Read the model definition and answer for the solid it produces. Units are mm, in the model's axes. Face numbers are marked on the shaded views. Coordinates: 2 decimals unless noted, no trailing zeros. Order: outer loops, then holes, each group sorted by start corner. A loop starts at its lowest first (then second) coordinate and runs counter-clockwise, first axis right, second up. Notation, with made-up numbers: (2.25, 43.25) -> (58.25, 43.25) arc R18 cw to (58.25, 75.25) -> close; hole circle Ø7 at (79, 65.25). An arc over 180 degrees is marked (long way). Answer as a JSON object with one key per item and string values. Group by question number.
1) Given pin 1 (3 mm diameter, centred on x = 16, y = 0, fed in from +Z); pin 2 (4 mm diameter, centred on x = -11.31, y = 11.31, fed in from -Z); pin 3 (4 mm diameter, centred on x = 17.5, z = 27.75, fed in from +Y); pin 4 (2.5 mm diameter, centred on x = -11.31, y = -11.31, fed in from +Z), each flat-ended and moving along its own axis, determine where each tip first touches the part or whether it passes through.
2) Consider L1, parallel to Y at x = 0, z = 19; L2, parallel to X at y = 12.5, z = 30; L3, parallel to X at y = 14, z = 26.5. Determine where each line is inside the solid, lowest interval first.
3) Determine the mould class of the marked faces 1, 2, 3 and 4 for opening direction X: released by +X, released by -X, zero draft, split by the parting line, or undercut.
4) Section B-B on y = 6.5 is taken. Count the separate pieces of the cut face and the enclosed holes in it, and give its area (3 significant figures).
5) Section A-A on z = 14.5 is taken. Determine the outline of the cut face in (x, y).
from build123d import *

# Parameters (mm, degrees)
ESQUISSE1_W               = 50
ESQUISSE1_H               = 36
BOSS_EXTRU_1_DEPTH        = 31.5
ESQUISSE2_R               = 11.25
ENL_V_MAT_EXTRU_1_DEPTH   = 31.5
TROU_TARAUD_M4X0_71_D     = 3.3
TROU_TARAUD_M4X0_71_DEPTH = 12
TROU_TARAUD_M4X0_71_TIP   = 0.991420021
TROU_TARAUD_M5X0_81_D     = 4.2
TROU_TARAUD_M5X0_81_DEPTH = 14
TROU_TARAUD_M5X0_81_TIP   = 1.2618073
CHANFREIN1_SIZE           = 1


with BuildPart() as part:
    # Esquisse1 → Boss.-Extru.1 (new body)
    with BuildSketch(Plane.XY):
        Rectangle(ESQUISSE1_W, ESQUISSE1_H)
    extrude(amount=BOSS_EXTRU_1_DEPTH)

    # Esquisse2 → Enlèv. mat.-Extru.1 (cut)
    with BuildSketch(Plane.XY.offset(31.5)):
        Circle(ESQUISSE2_R)
    extrude(amount=-ENL_V_MAT_EXTRU_1_DEPTH, mode=Mode.SUBTRACT)

    # Trou taraudé M4x0.71
    with Locations(Plane.XY.offset(31.5)):
        with Locations((-11.313708499, 11.313708499), (-16, 0), (-11.313708499, -11.313708499), (11.313708499, -11.313708499), (16, 0), (11.313708499, 11.313708499)):
            Hole(TROU_TARAUD_M4X0_71_D / 2, depth=TROU_TARAUD_M4X0_71_DEPTH)
            with Locations((0, 0, -(TROU_TARAUD_M4X0_71_DEPTH + TROU_TARAUD_M4X0_71_TIP / 2))):  # 118° drill point
                Cone(0, TROU_TARAUD_M4X0_71_D / 2, TROU_TARAUD_M4X0_71_TIP, mode=Mode.SUBTRACT)

    # Trou taraudé M5x0.81
    with Locations(Plane(origin=(0, 18, 0), x_dir=(1, 0, 0), z_dir=(0, 1, 0))):
        with Locations((-17.5, -27.75), (-17.5, -3.75), (17.5, -3.75), (17.5, -27.75)):
            Hole(TROU_TARAUD_M5X0_81_D / 2, depth=TROU_TARAUD_M5X0_81_DEPTH)
            with Locations((0, 0, -(TROU_TARAUD_M5X0_81_DEPTH + TROU_TARAUD_M5X0_81_TIP / 2))):  # 118° drill point
                Cone(0, TROU_TARAUD_M5X0_81_D / 2, TROU_TARAUD_M5X0_81_TIP, mode=Mode.SUBTRACT)

    # Chanfrein1
    chanfrein1_edges = [part.edges().sort_by_distance(p)[0] for p in [
        (-11.25, 0, 0),
        (-11.25, 0, 31.5),
    ]]
    chamfer(chanfrein1_edges, length=CHANFREIN1_SIZE)


solid = part.part
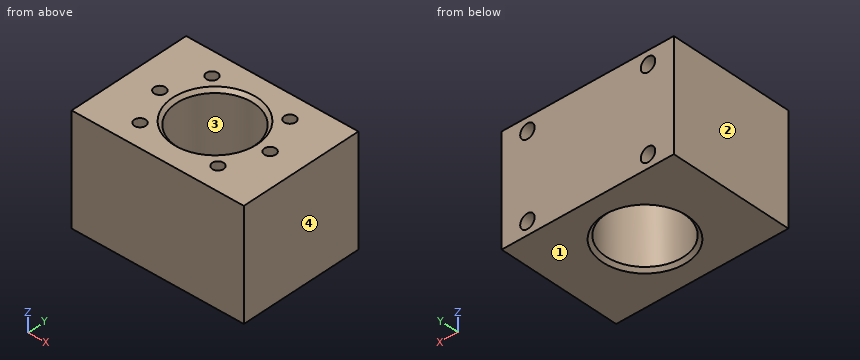
Worked answers:
{
 "1": {"pin 1": "stops at z = 19.41", "pin 2": "stops at z = 0", "pin 3": "stops at y = 3.94", "pin 4": "stops at z = 19.26"},
 "2": {"L1": "y = -18 to -11.25, 11.25 to 18", "L2": "x = -25 to -12.46, -10.17 to 10.17, 12.46 to 25", "L3": "x = -25 to -19.19, -15.81 to 15.81, 19.19 to 25"},
 "3": {"face 1": "zero draft", "face 2": "released by -X", "face 3": "undercut", "face 4": "released by +X"},
 "4": {"separate pieces": "2", "enclosed holes": "4", "area": "939 mm²"},
 "5": {"outline": "(-25, -18) -> (25, -18) -> (25, 18) -> (-25, 18) -> close; hole circle Ø22.5 at (0, 0)"}
}
